Could you check a few things on this model? Use its own coordinates, in mm. A direction names the side the tool comes from. Coordinates: 2 decimals unless noted, no trailing zeros. Write each loop counter-clockwise with the first axis right and the second up, starting at its lowest first coordinate (ties: lowest second). Pieces come first, ordered by that corner, then holes. Notation, with made-up numbers: M 7,-9 L 55,-9 A20 cw 55,15 Z; hole C -26,75 d7. An arc over 180 degrees is marked long. Write item = value, one per line.
Autodesk Inventor part; units mm, degrees
ref_plane "YZ Plane" through (0, 0, 0) normal (1, 0, 0) x (0, 1, 0)
ref_plane "XZ Plane" through (0, 0, 0) normal (0, 1, 0) x (-1, 0, 0)
ref_plane "XY Plane" through (0, 0, 0) normal (0, 0, 1) x (1, 0, 0)
sketch "Эскиз1" plane through (0, 0, 0) normal (0, 0, 1) x (1, 0, 0)
  line L0 (-1.4, 0) -> (-1.4, -14.4)
  line L1 (-1.4, -14.4) -> (0, -14.4)
  line L2 (0, -14.4) -> (0, 1.6)
  line L3 (0, 1.6) -> (-2.8, 1.6)
  line L4 (-2.8, 1.6) -> (-2.8, 1.4)
  line L5 (-2.8, 1.4) -> (-1.4, 0)
  point P0 (0, 0)
  dimension "d0" = 2.8
  dimension "d2" = 45
  dimension "d3" = 1.6
  dimension "d4" = 16
  dimension "d5" = 5.6
revolve "Вращение1" add sketch "Эскиз1" angle 360 about axis through (0, -14.4, 0) along (0, 1, 0)
sketch "Эскиз2" plane through (0, 0, 0) normal (1, 0, 0) x (0, 1, 0)
  line L0 (1.6, -2.8) -> (1.6, 2.8)
  line L1 (1.6, 1.5) -> (1.6, 0)
  line L2 (0, 0) -> (1.6, 0)
  line L3 (1.6, 1.5) -> (0, 0.5)
  line L4 (0, -1.4) -> (0, 1.4)
  line L5 (0, 0) -> (0, 0.5)
  dimension "d7" = 1.5
  dimension "d13" = 0.5
extrude "Выдавливание1" cut sketch "Эскиз2" along normal mid plane 1
pattern_circular "Круговой массив1" count 4 over 360 about axis through (0, -10, 0) along (0, 1, 0) of "Выдавливание1"
thread "Резьба1"
properties part number "M3x10P"
Item 1: Imagine slicing it at C-C (y = -6.5). Write out the boundary of the cut face in (x, z).
Numbers:
outline = C 0,0 d2.8
Item 2: If we mould it in two halves opening along X, with no side actions, what happens to faces 3 (the face through (-1, 1.6, -1)), 4 (the face through (1.4, -7.3, -0.06)), 5 (the face through (0.5, 1.1, -0.8))? For each: pulls with the +X half, pulls with the -X half, needs draft (parallel to the pull), parting line crosses it, or undercut.
Numbers:
face_3 = needs draft
face_4 = parting line crosses it
face_5 = undercut
Item 3: If I drill on line 1 along X through (y, z) = (-0.5, 0.1); line 2 along Y through (x, z) = (-2, -0.2); line 3 along Y through (x, z) = (2.25, 0.3), over which ranges is the centre line in solid material (lowest first)?
Numbers:
line_1 = -1.4 to 1.4
line_2 = 0.61 to 1.6
line_3 = 0.87 to 1.6
Item 4: For faces 1 (the face through (0, -14.4, 0)), 2 (the face through (0, 0.8, -1)), which set-ups out of +Z, -Z, +X, -X, +Y, -Y let a thin tool reach every point of the face, with its end or its side?
Numbers:
face_1 = +Z, -Z, +X, -X, -Y
face_2 = +Y
Item 5: Imagine slicing it at B-B (z = 0). Write out the boundary of the cut face in (x, y).
Numbers:
outline = M -2.8,1.4 L -1.4,0 L -1.4,-14.4 L 1.4,-14.4 L 1.4,0 L 2.8,1.4 L 2.8,1.6 L 1.5,1.6 L 0.5,0 L -0.5,0 L -1.5,1.6 L -2.8,1.6 Z
Item 6: I'm going to push flat-ended pins straight in: P1, Ø0.5, axis at x = 1, y = 1, coming from the +Z side; P2, Ø1.1, axis at x = -1, y = 0.5, coming from the +Z side; P3, Ø1.1, axis at y = 1, z = -1, coming from the -X side. Where does each tip first touch, or does it pass through?
Numbers:
P1 = 2.47
P2 = 2.28
P3 = -2.73
Item 7: Imagine slicing it at A-A (x = 0). Write out the boundary of the cut face in (y, z).
Numbers:
outline = M -14.4,-1.4 L 0,-1.4 L 1.4,-2.8 L 1.6,-2.8 L 1.6,-1.5 L 0,-0.5 L 0,0.5 L 1.6,1.5 L 1.6,2.8 L 1.4,2.8 L 0,1.4 L -14.4,1.4 Z
